Here's the drawing with two shaded views (mm, measured from the low corner). I have some questions. A direction names the side the tool comes from. Give positions to 0.01 mm unless a question says otherwise; leave off trailing zeros. Loops run counter-clockwise (first coordinate to the right, second up) from the corner with the lowest first, then second, coordinate; pieces in that order, holes last. Notation, with made-up numbers: (15.25, -36.75) - (56.25, -36.75) arc R13 cw to (56.25, -12.75) - close; hole circle Ø1 at (-26.75, -9.75). An arc over 180 degrees is marked (long way). Answer as a JSON object with one key per item and string values. Group by question number.
Item 1: Thinking about a two-plate mould opening in Z: for the marked faces 1, 2, 3 and 4, which applies, pulls with the +Z half, pulls with the -Z half, needs draft (parallel to the pull), parting line crosses it, or undercut?
Item 2: Suppose I cut it at C-C on x = 7.5. Write out the boundary of the cut face in (y, z), and give its area (3 significant figures).
Item 3: Please list where these lines run through material, in increasing order: L1, parallel to X at y = 7, z = 29.3; L2, parallel to Y at x = 20, z = 29; L3, parallel to Z at x = 24.5, y = 5.5.
Item 4: Will these pins go through, and if not, where does the flat tip stop? pin 1 (0.7 mm diameter, centred on y = 6.5, z = 29.5, fed in from +X); pin 2 (4.5 mm diameter, centred on x = 1.8, y = 7, fed in from +Z); pin 3 (5 mm diameter, centred on y = 11.5, z = 12.5, fed in from +X).
Item 5: Suppose I cut it at B-B on z = 17.5. Write out the boundary of the cut face in (x, y), and give its area (3 significant figures).
Item 6: Which directions (+Z, -Z, +X, -X, +Y, -Y) give clear straight access to the entire face, cutting with the end or side of a thin tool? Please do the marked faces 5, 6, 7, 8 and 9.
Item 7: Suppose I cut it at D-D on y = 1. Write out the boundary of the cut face in (x, z).
Item 8: Suppose I cut it at A-A on x = 31.8. Write out the boundary of the cut face in (y, z).
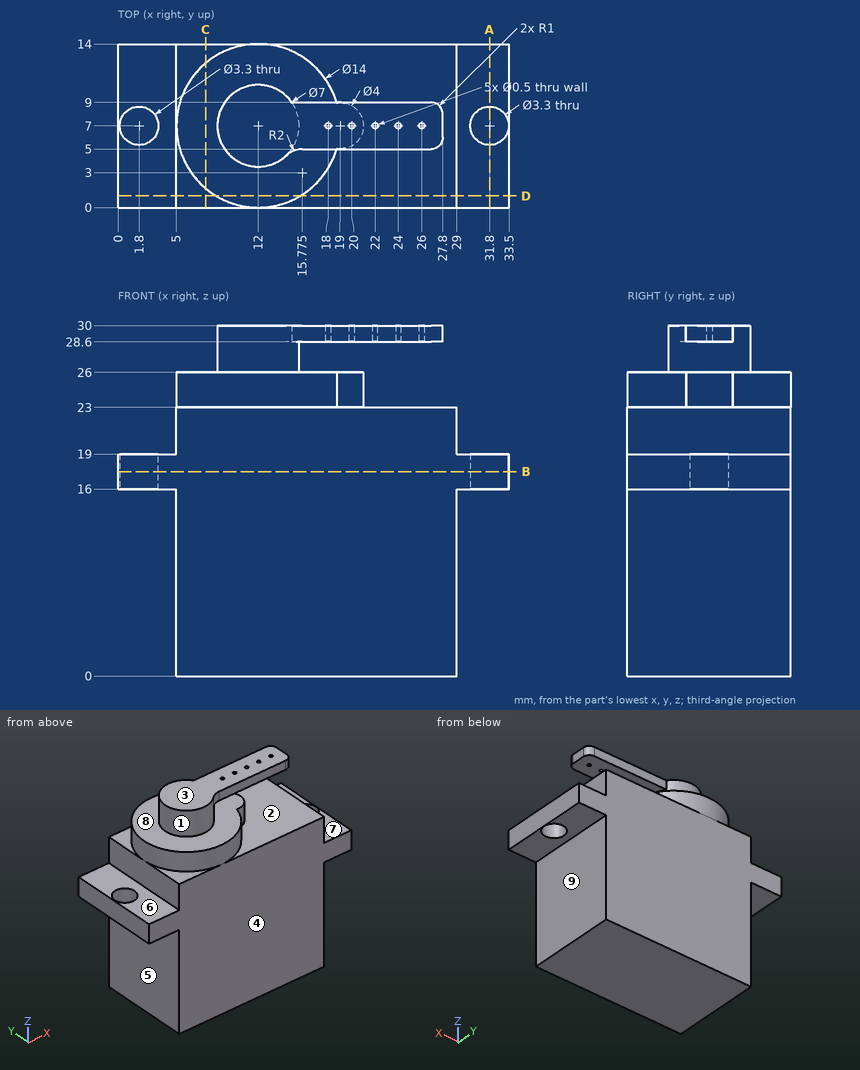
Worked out:
{
 "1": {"face 1": "undercut", "face 2": "undercut", "face 3": "pulls with the +Z half", "face 4": "needs draft"},
 "2": {"outline": "(0, 0) - (14, 0) - (14, 23) - (12.36, 23) - (12.36, 26) - (1.64, 26) - (1.64, 23) - (0, 23) - close", "area": "354 mm2"},
 "3": {"L1": "x = 8.5 to 17.75, 18.25 to 19.75, 20.25 to 21.75, 22.25 to 23.75, 24.25 to 25.75, 26.25 to 27.8", "L2": "y = 5 to 6.75, 7.25 to 9", "L3": "z = 0 to 23, 28.6 to 30"},
 "4": {"pin 1": "stops at x = 27.8", "pin 2": "stops at z = 19", "pin 3": "stops at x = 29"},
 "5": {"outline": "(0, 0) - (33.5, 0) - (33.5, 14) - (0, 14) - close; hole circle Ø3.3 at (1.8, 7); hole circle Ø3.3 at (31.8, 7)", "area": "452 mm2"},
 "6": {"face 5": "-Z, -X, +Y, -Y", "face 6": "+Z, -X, +Y, -Y", "face 7": "+Z, +X, +Y, -Y", "face 8": "none", "face 9": "-Z, +X, +Y, -Y"},
 "7": {"outline": "(0, 16) - (5, 16) - (5, 0) - (29, 0) - (29, 16) - (33.5, 16) - (33.5, 19) - (29, 19) - (29, 23) - (15.61, 23) - (15.61, 26) - (8.39, 26) - (8.39, 23) - (5, 23) - (5, 19) - (0, 19) - close"},
 "8": {"outline": "(0, 16) - (5.35, 16) - (5.35, 19) - (0, 19) - close; (8.65, 16) - (14, 16) - (14, 19) - (8.65, 19) - close"}
}
